from build123d import *

# Parameters (mm, degrees)
SKETCH1_R           = 3.048
BOSS_EXTRUDE2_DEPTH = 6.35


with BuildPart() as part:
    # Sketch1 → Boss-Extrude2 (new body)
    with BuildSketch(Plane.XY):
        with BuildLine():
            ThreePointArc((-19.685, 0), (-19.36354027, 3.542955436), (-18.409660074, 6.970196624))
            Line((-18.409660074, 6.970196624), (-34.253888671, 26.312396902))
            Line((-34.253888671, 26.312396902), (-39.107436935, 26.312396902))
            ThreePointArc((-39.107436935, 26.312396902), (-40.005462547, 25.940422514), (-40.377436935, 25.042396902))
            Line((-40.377436935, 25.042396902), (-40.377436935, -58.42))
            ThreePointArc((-40.377436935, -58.42), (-40.005462547, -59.318025612), (-39.107436935, -59.69))
            Line((-39.107436935, -59.69), (-19.685, -59.69))
            Line((-19.685, -59.69), (-19.685, 0))
        make_face()
        with Locations((-30.382536935, 7.262396902)):
            Circle(SKETCH1_R, mode=Mode.SUBTRACT)
        with Locations((-30.382536935, -45.72)):
            Circle(SKETCH1_R, mode=Mode.SUBTRACT)
    extrude(amount=BOSS_EXTRUDE2_DEPTH)


solid = part.part
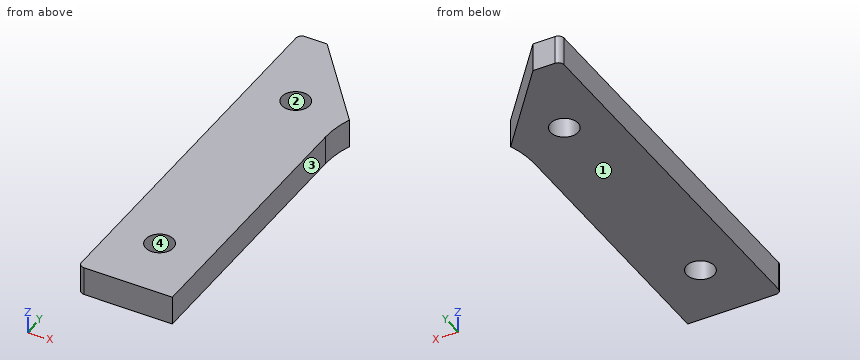
Input: part model. Units: mm. Frame: model coordinates. Face numbers are marked on the shaded views. Coordinates: 2 decimals unless noted, no trailing zeros. Write each loop counter-clockwise with the first axis right and the second up, starting at its lowest first coordinate (ties: lowest second). Pieces come first, ordered by that corner, then holes. Notation, with made-up numbers: M -37.75,55 L 5.25,55 A12 ccw 5.25,69 Z; hole C 24.5,-26.75 d5. An arc over 180 degrees is marked long. Answer as a JSON object with one key per item and string values. Group by question number.
(1) Section C-C on z = 3.5. Output: boundary loops of the cut face in (x, y) (3 decimals).
(2) Section A-A on y = -45.72. Output: boundary loops of the cut face in (x, z) (3 decimals).
(3) Section B-B on x = -29.75. Output: boundary loops of the cut face in (y, z).
(4) Ray query, line 1 along Y through (x, z) = (-31, 1.25); line 2 along X through (y, z) = (-49.5, 4.25) (3 decimals); line 3 along Y through (x, z) = (-34.25, 3). Return the intervals inside material, ascending. Write a range as [from, to].
(5) Mould query, pull axis X, two halves, no side actions, for the marked faces 1, 2, 3 and 4. Classes: pulls with the +X half, pulls with the -X half, needs draft (parallel to the pull), parting line crosses it, or undercut.
(6) Section D-D on y = -16. Output: boundary loops of the cut face in (x, z) (3 decimals), plus the area to 3 significant figures.
(7) Contact query for a flat-ended pin moving along its axis: P1, Ø3, axis at y = -32, z = 3, coming from the +X side (3 decimals). Output: stop coordinate, or through.
Result set:
{
 "1": {"outline": "M -40.377,-58.42 A1.27 ccw -39.107,-59.69 L -19.685,-59.69 L -19.685,0 A19.685 cw -18.41,6.97 L -34.254,26.312 L -39.107,26.312 A1.27 ccw -40.377,25.042 Z; hole C -30.383,-45.72 d6.096; hole C -30.383,7.262 d6.096"},
 "2": {"outline": "M -40.377,0 L -33.431,0 L -33.431,6.35 L -40.377,6.35 Z; M -27.335,0 L -19.685,0 L -19.685,6.35 L -27.335,6.35 Z"},
 "3": {"outline": "M -59.69,0 L -48.7,0 L -48.7,6.35 L -59.69,6.35 Z; M -42.74,0 L 4.28,0 L 4.28,6.35 L -42.74,6.35 Z; M 10.24,0 L 20.81,0 L 20.81,6.35 L 10.24,6.35 Z"},
 "4": {"line 1": "y = [-59.69, -48.7], [-42.74, 4.28], [10.25, 22.34]", "line 2": "x = [-40.377, -19.685]", "line 3": "y = [-59.69, 26.31]"},
 "5": {"face 1": "needs draft", "face 2": "undercut", "face 3": "pulls with the +X half", "face 4": "undercut"},
 "6": {"outline": "M -40.377,0 L -19.685,0 L -19.685,6.35 L -40.377,6.35 Z", "area": "131 mm2"},
 "7": {"P1": "stops at x = -19.685"}
}
